Autodesk Inventor part; units mm, degrees
ref_plane "Work Plane1" through (54.1997, -954.1849, -9.0948) normal (0, 0, 1) x (0.9638, -0.2666, 0)
ref_plane "YZ Plane" through (0, 0, 0) normal (1, 0, 0) x (0, 1, 0)
ref_plane "XZ Plane" through (0, 0, 0) normal (0, 1, 0) x (-1, 0, 0)
sketch "Sketch1" plane through (0, 0, 0) normal (0, 0, 1) x (1, 0, 0)
  line L0 (0, -1000) -> (0, -848) construction
  line L1 (-15, -848) -> (-15, -1000) construction
  line L2 (-15, -963.9285) -> (0, -963.9285)
  line L3 (0, -963.9285) -> (0, -908.9285)
  line L4 (0, -908.9285) -> (-15, -908.9285)
  line L5 (-15, -908.9285) -> (-15, -963.9285)
  line L6 (0, -963.9285) -> (3, -963.9285)
  line L7 (3, -963.9285) -> (3, -908.9285)
  line L8 (3, -908.9285) -> (0, -908.9285)
  line L9 (0, -908.9285) -> (0, -963.9285)
  line L10 (-7.5, -908.9285) -> (-7.5, -963.9285) construction
  circle A0 centre (-7.5, -922.6785) radius 1.7
  circle A1 centre (-7.5, -936.4285) radius 1.7
  circle A2 centre (-7.5, -950.1785) radius 1.7
  line L11 (-15, -936.4285) -> (3, -936.4285) construction
  point P0 (0, 0)
  dimension "d6" = 55
  dimension "d7" = 3
  dimension "d22" = 3.4
  dimension "d23" = 3.4
  dimension "d24" = 3.4
  dimension "d25" = 13.75
  dimension "d26" = 13.75
extrude "Extrusion1" add sketch "Sketch1" along normal blind 3
sketch "Sketch2" plane through (0, 0, 0) normal (0, 0, -1) x (-1, 0, 0)
  line L0 (-3, -963.9285) -> (-3, -908.9285)
  line L1 (-3, -908.9285) -> (15, -908.9285)
  line L2 (-3, -963.9285) -> (0, -963.9285)
  line L3 (0, -963.9285) -> (0, -908.9285)
  line L4 (0, -908.9285) -> (-3, -908.9285)
  line L5 (-3, -908.9285) -> (-3, -963.9285)
  point P0 (0, 0)
ref_plane "Work Plane1" through (54.1997, -954.1849, -9.0948) normal (0, 0, 1) x (0.9638, -0.2666, 0)
extrude "Extrusion2" add sketch "Sketch2" along normal up to surface (9.0948 mm away)
sketch "Sketch3" plane through (3, -963.9285, -9.0948) normal (0, 0, -1) x (-1, 0, 0)
  line L0 (0, 0) -> (0, 55)
  line L1 (0, 27.5) -> (-10, 27.5) construction
  line L2 (-20, 7.5) -> (0, 7.5)
  line L3 (0, 7.5) -> (0, 47.5)
  line L4 (0, 47.5) -> (-20, 47.5)
  line L5 (-20, 47.5) -> (-20, 7.5)
  line L6 (-20, 7.5) -> (0, 47.5) construction
  line L7 (0, 7.5) -> (-20, 47.5) construction
  line L8 (-14.95, 3.5) -> (-5.05, 3.5) construction
  line L9 (-5.05, 3.5) -> (-5.05, 51.5) construction
  line L10 (-5.05, 51.5) -> (-14.95, 51.5) construction
  line L11 (-14.95, 51.5) -> (-14.95, 3.5) construction
  line L12 (-14.95, 3.5) -> (-5.05, 51.5) construction
  line L13 (-5.05, 3.5) -> (-14.95, 51.5) construction
  circle A0 centre (-14.95, 3.5) radius 1.7
  line L14 (-10, 3.5) -> (-10, 51.5) construction
  circle A1 centre (-14.95, 51.5) radius 1.7
  circle A2 centre (-5.05, 3.5) radius 1.7
  circle A3 centre (-5.05, 51.5) radius 1.7
  line L15 (3, 0) -> (-21, 0)
  line L16 (-23, 2) -> (-23, 53)
  line L17 (-21, 55) -> (3, 55)
  line L18 (3, 55) -> (3, 0)
  line L19 (3, 0) -> (-23, 55) construction
  line L20 (-23, 0) -> (3, 55) construction
  arc A4 (-23, 2) -> (-21, 0) centre (-21, 2) ccw
  arc A5 (-21, 55) -> (-23, 53) centre (-21, 53) ccw
  point P0 (3, 963.9285)
  point P1 (0, 7.5)
  dimension "d12" = 10
  dimension "d13" = 40
  dimension "d14" = 9.9
  dimension "d15" = 48
  dimension "d16" = 3.4
  dimension "d17" = 26
  dimension "d18" = 55
  dimension "d19" = 2
extrude "Extrusion3" add sketch "Sketch3" against normal blind 3 contours L15 A4 L16 A5 L17 L0 L4 L5 L2 | L0 L17 L18 L15
properties part number "ServoMount"
Input: part model. Units: mm. Frame: model coordinates. A direction names the side the tool comes from. Coordinates: 2 decimals unless noted, no trailing zeros. Order: outer loops, then holes, each group sorted by start corner. A loop starts at its lowest first (then second) coordinate and runs counter-clockwise, first axis right, second up. Notation, with made-up numbers: M 25,82.5 L 39,82.5 A10 ccw 39,91.5 Z; hole C -21,-5 d11. An arc over 180 degrees is marked long. Answer as CSV lines item,"result".
1. First-contact query: P1, Ø5, axis at x = -6.5, z = -2, coming from the +Y side; P2, Ø4, axis at x = 17.95, y = -912.43, coming from the +Z side; P3, Ø0.9, axis at y = -941, z = -8, coming from the -X side; P4, Ø1, axis at x = -6, z = -2, coming from the +Y side. Flat tips, straight axial feed; report the tip coordinate or a pass-through.
Reported:
P1,"y = -908.93"
P2,"z = -6.09"
P3,"x = 0"
P4,"through"
2. Pull-direction query (X, two-part tool) for faces 1 (the flat face through (-9.3, -936, 0)), 2 (the cylindrical face through (25.43, -963.327, -7.616)), 3 (the cylindrical face through (17.17, -913.94, -7.62)); classes: released by +X, released by -X, zero draft, split by the parting line, or undercut.
Reported:
face 1,"zero draft"
face 2,"released by +X"
face 3,"undercut"
3. Access query for faces 4 (the flat face through (3, -937, -3)), 5 (the flat face through (13, -916.428, -8)), 6 (the flat face through (24, -936, -6.095)), 7 (the flat face through (0, -937, -4)). Directions: +Z, -Z, +X, -X, +Y, -Y. A direction counts if a zero-diameter tool reaches every point of the face in a straight line with its end or side. Return the directions, or none.
Reported:
face 4,"+Z"
face 5,"+Z, -Z"
face 6,"+Z, +X, +Y, -Y"
face 7,"-Z, -X, +Y, -Y"
4. Section C-C (z = 1.5). Return the cut outline in (x, y).
Reported:
outline,"M -15,-963.93 L 3,-963.93 L 3,-908.93 L -15,-908.93 Z; hole C -7.5,-950.18 d3.4; hole C -7.5,-936.43 d3.4; hole C -7.5,-922.68 d3.4"
5. Material intervals for line 1 (Y direction, x = 8, z = -7.75); line 2 (Y direction, x = 4.5, z = -7.75); line 3 (X direction, y = -926, z = -6.25), sorted ascending. Write a range as from..to.
Reported:
line 1,"-963.93..-962.13, -958.73..-956.43, -916.43..-914.13, -910.73..-908.93"
line 2,"-963.93..-956.43, -916.43..-908.93"
line 3,"0..3, 23..26"
6. Section A-A (x = 8.05). Return the cut outline in (y, z).
Reported:
outline,"M -963.93,-9.09 L -962.13,-9.09 L -962.13,-6.09 L -963.93,-6.09 Z; M -958.73,-9.09 L -956.43,-9.09 L -956.43,-6.09 L -958.73,-6.09 Z; M -916.43,-9.09 L -914.13,-9.09 L -914.13,-6.09 L -916.43,-6.09 Z; M -910.73,-9.09 L -908.93,-9.09 L -908.93,-6.09 L -910.73,-6.09 Z"
7. Section D-D (x = -7.5). Return the cut outline in (y, z).
Reported:
outline,"M -963.93,0 L -951.88,0 L -951.88,3 L -963.93,3 Z; M -948.48,0 L -938.13,0 L -938.13,3 L -948.48,3 Z; M -934.73,0 L -924.38,0 L -924.38,3 L -934.73,3 Z; M -920.98,0 L -908.93,0 L -908.93,3 L -920.98,3 Z"
8. Section B-B (y = -922). Return the cut outline in (x, z), then the cut area to 3 significant figures.
Reported:
outline,"M -15,0 L -9.06,0 L -9.06,3 L -15,3 Z; M -5.94,0 L 0,0 L 0,-9.09 L 3,-9.09 L 3,3 L -5.94,3 Z; M 23,-9.09 L 26,-9.09 L 26,-6.09 L 23,-6.09 Z"
area,"80.9 mm2"
